Geometry check sheet. Reference: the model listing, model coordinates, mm. A direction names the side the tool comes from. Round coordinates to 2 decimals unless told otherwise and drop trailing zeros. Write each loop counter-clockwise with the first axis right and the second up, starting at its lowest first coordinate (ties: lowest second). Pieces come first, ordered by that corner, then holes. Notation, with made-up numbers: (70.25, 22) - (125.25, 22) arc R34 cw to (125.25, 60) - close; hole circle Ø4 at (39.5, -37). An arc over 180 degrees is marked (long way). Return JSON: item names as keys, results as strings.
```python
from build123d import *

# Parameters (mm, degrees)
LUGGAP_DEPTH    = 6.35
LUGGAPPAT_COUNT = 3


with BuildPart() as part:
    # BodySke → Body (revolve)
    with BuildSketch(Plane.XY, mode=Mode.PRIVATE) as body_sk:
        with BuildLine():
            Line((4.0005, 0), (4.8674655, 0))
            Line((4.8674655, 0), (5.7370345, -0.6096))
            Line((5.7370345, -0.6096), (6.604, 0))
            Line((6.604, 0), (6.604, 4.318))
            ThreePointArc((6.604, 4.318), (6.492407684, 4.587407684), (6.223, 4.699))
            Line((6.223, 4.699), (2.5527, 4.699))
            Line((2.5527, 4.699), (2.5527, -1.2192))
            Line((2.5527, -1.2192), (4.0005, -1.2192))
            Line((4.0005, -1.2192), (4.0005, 0))
        make_face()
    revolve(body_sk.sketch.rotate(Axis((0, 4.318, 0), (0, 1, 0)), 90), axis=Axis((0, 4.318, 0), (0, 1, 0)))

    # EndChamferSke → EndChamfer (revolve, cut)
    with BuildSketch(Plane.XY, mode=Mode.PRIVATE) as endchamfer_sk:
        Polygon((3.175, -1.4732), (3.175, -0.9652), (2.5527, -0.529622692), (2.5527, -1.4732), align=None)
        Polygon((3.175, 4.699), (2.5527, 4.263422692), (2.5527, 4.699), align=None)
    revolve(endchamfer_sk.sketch.rotate(Axis((0, -2.54, 0), (0, 1, 0)), 90), axis=Axis((0, -2.54, 0), (0, 1, 0)), mode=Mode.SUBTRACT)

    # LugGapSke → LugGap (cut)
    with BuildSketch(Plane(origin=(0, 0, 0), x_dir=(1, 0, 0), z_dir=(0, 1, 0))):
        with BuildLine():
            Line((-0.925840238, -4.778602332), (-1.830362504, -6.345280853))
            ThreePointArc((-1.830362504, -6.345280853), (3.302, -5.719231767), (6.410355665, -1.5875))
            Line((6.410355665, -1.5875), (4.601311133, -1.5875))
            ThreePointArc((4.601311133, -1.5875), (2.43373275, -4.215348775), (-0.925840238, -4.778602332))
        make_face()
    luggap = extrude(amount=-LUGGAP_DEPTH, mode=Mode.SUBTRACT)

    # LugGapPat: LugGap ×3 about axis
    luggappat_axis = Axis((0, 0, 0), (0, 1, 0))
    for i in range(1, LUGGAPPAT_COUNT):
        add(luggap.rotate(luggappat_axis, i * 360 / LUGGAPPAT_COUNT), mode=Mode.SUBTRACT)


solid = part.part
```
(1) Release check for a two-part mould opening along Z. For faces 1 (the face through (-0.767, 1.833, -2.435)), 2 (the face through (-3.06, -0.37, 5.25)), 3 (the face through (-1.98, 2.19, -6.3)) record: pulls with the +Z half, pulls with the -Z half, needs draft (parallel to the pull), parting line crosses it, or undercut.
Response values:
{"face 1": "undercut", "face 2": "pulls with the +Z half", "face 3": "parting line crosses it"}
(2) Material ranges on line 1 along X through (y, z) = (0.6, 0); line 2 along X through (y, z) = (-1.1, 0) (1 decimal); line 3 along Y through (x, z) = (-1, 4), recorded low to high. Write a range as [from, to].
Response values:
{"line 1": "x = [-6.6, -2.55], [2.55, 6.6]", "line 2": "x = [-4, -3.2], [3.2, 4]", "line 3": "y = [0, 4.7]"}
(3) Access from +Z, -Z, +X, -X, +Y, -Y to the whole of each face (thin tool, end or side, straight path). Record for faces 4 (the face through (-2.58, -0.24, -4.53)), 5 (the face through (-1.4, -0.2, 5.6)), 6 (the face through (-4.134, -0.233, 3.985)), 7 (the face through (-1.4, -0.2, -5.6)).
Response values:
{"face 4": "-Y", "face 5": "+Z, +X, -Y", "face 6": "-X, -Y", "face 7": "-Z, +X, -Y"}
(4) Gauge pin test, flat ends, axial feed: pin 1 (1.5 mm diameter, centred on y = 0.5, z = 5, fed in from +X); pin 2 (1 mm diameter, centred on y = 1.5, z = 5, fed in from +X); pin 3 (3 mm diameter, centred on y = 3.5, z = 2, fed in from +X). Record the tip position at first contact, or that the pin passes through.
Response values:
{"pin 1": "stops at x = 5.05", "pin 2": "stops at x = 4.83", "pin 3": "stops at x = 6.59"}
(5) Section check C-C, the plane y = 3.35. Enter the section's corners in (x, z).
Response values:
{"outline": "circle Ø13.21 at (0, 0); hole circle Ø5.11 at (0, 0)"}
